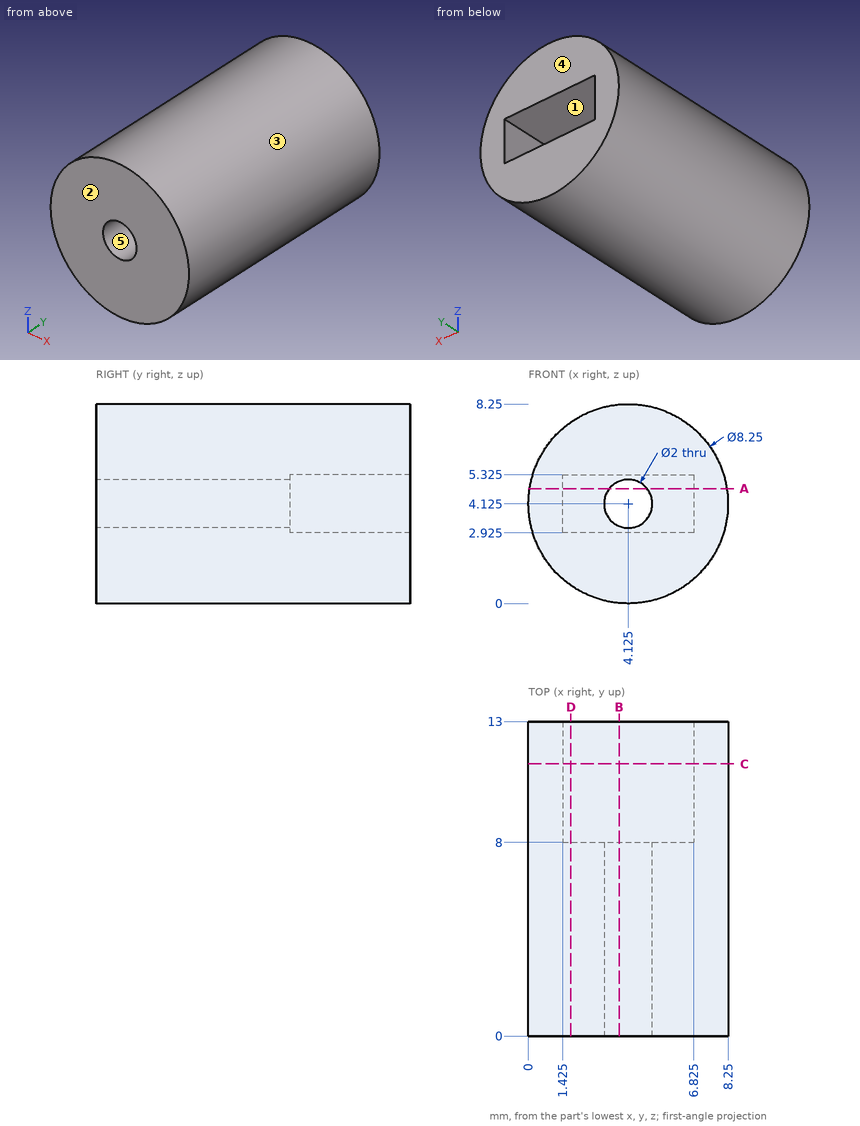
Geometry check sheet. Reference: drawing and pictorial views, mm from the part's lowest x, y, z. A direction names the side the tool comes from. Coordinates: 2 decimals unless noted, no trailing zeros. Order: outer loops, then holes, each group sorted by start corner. A loop starts at its lowest first (then second) coordinate and runs counter-clockwise, first axis right, second up. Notation, with made-up numbers: M 59,12 L 96,12 A11 cw 96,17 Z; hole C -26,19 d2. An arc over 180 degrees is marked long. Write each question's results on one line, items separated by ' | '. Start each with the question number.
1. Access from +Z, -Z, +X, -X, +Y, -Y to the whole of each face (thin tool, end or side, straight path). Record for the marked faces 1 and 2.
2. Cross-section at D-D on x = 1.75. Record the cut outline in (y, z) (3 decimals), and give its area (3 significant figures).
3. Mould release check, pull along X, two halves, no side actions. Record for the marked faces 3, 4 and 5: +X half, -X half, draft (parallel to the pull), parting line (faces both ways), or undercut.
4. Cross-section at C-C on y = 11.25. Record the cut outline in (x, z) (3 decimals).
5. Cross-section at A-A on z = 4.75. Record the cut outline in (x, y) (3 decimals), and give its area (3 significant figures).
6. Material ranges on probe 1 along X at (y, z) = (8.25, 4.25) (3 decimals); probe 2 along Z at (x, y) = (4, 8.5) (3 decimals); probe 3 along X at (y, z) = (2.25, 3.75), recorded low to high.
7. Cross-section at B-B on x = 3.75. Record the cut outline in (y, z) (3 decimals).
8. Go/stop test with flat-tipped pins: P1, Ø3, axis at y = 5, z = 6.5, coming from the +X side; P2, Ø1, axis at y = 6, z = 2, coming from the +X side; P3, Ø1, axis at y = 10.5, z = 6, coming from the -X side. Record where each tip stops, or that it passes through.
Checks:
1) face 1: +Y | face 2: +Z, -Z, +X, -X, -Y
2) outline: M 0,0.752 L 13,0.752 L 13,2.925 L 8,2.925 L 8,5.325 L 13,5.325 L 13,7.498 L 0,7.498 Z | area: 75.7 mm²
3) face 3: parting line | face 4: draft | face 5: undercut
4) outline: C 4.125,4.125 d8.25; hole M 1.425,2.925 L 6.825,2.925 L 6.825,5.325 L 1.425,5.325 Z
5) outline: M 0.048,0 L 3.344,0 L 3.344,8 L 1.425,8 L 1.425,13 L 0.048,13 Z; M 4.906,0 L 8.202,0 L 8.202,13 L 6.825,13 L 6.825,8 L 4.906,8 Z | area: 66.5 mm²
6) probe 1: x = 0.002 to 1.425, 6.825 to 8.248 | probe 2: z = 0.002 to 2.925, 5.325 to 8.248 | probe 3: x = 0.02 to 3.2, 5.05 to 8.23
7) outline: M 0,0.017 L 13,0.017 L 13,2.925 L 8,2.925 L 8,3.198 L 0,3.198 Z; M 0,5.052 L 8,5.052 L 8,5.325 L 13,5.325 L 13,8.233 L 0,8.233 Z
8) P1: stops at x = 8.16 | P2: stops at x = 7.92 | P3: stops at x = 0.24
